```python
from build123d import *

# Parameters (mm, degrees)
SKETCH1_W                 = 175
SKETCH1_H                 = 110
BOSS_EXTRUDE1_DEPTH       = 10
SKETCH3_W                 = 30
SKETCH3_H                 = 15
BOSS_EXTRUDE2_DEPTH       = 40
M3X0_5_TAPPED_HOLE1_D     = 2.5
M3X0_5_TAPPED_HOLE1_DEPTH = 7.5
M3X0_5_TAPPED_HOLE1_TIP   = 0.751075774


with BuildPart() as part:
    # Sketch1 → Boss-Extrude1 (new body)
    with BuildSketch(Plane(origin=(0, 0, 0), x_dir=(1, 0, 0), z_dir=(0, 1, 0))):
        with Locations((87.5, 55)):
            Rectangle(SKETCH1_W, SKETCH1_H)
    extrude(amount=BOSS_EXTRUDE1_DEPTH)

    # Sketch3 → Boss-Extrude2 (add)
    with BuildSketch(Plane(origin=(0, 10, 0), x_dir=(1, 0, 0), z_dir=(0, 1, 0))):
        with Locations((55, 7.5)):
            Rectangle(SKETCH3_W, SKETCH3_H)
        with Locations((55, 102.5)):
            Rectangle(SKETCH3_W, SKETCH3_H)
    extrude(amount=BOSS_EXTRUDE2_DEPTH)

    # M3x0.5 Tapped Hole1
    with Locations(Plane(origin=(0, 50, 0), x_dir=(-1, 0, 0), z_dir=(0, 1, 0))):
        with Locations((-45, -7.5), (-65, -7.5), (-45, -102.5), (-65, -102.5)):
            Hole(M3X0_5_TAPPED_HOLE1_D / 2, depth=M3X0_5_TAPPED_HOLE1_DEPTH)
            with Locations((0, 0, -(M3X0_5_TAPPED_HOLE1_DEPTH + M3X0_5_TAPPED_HOLE1_TIP / 2))):  # 118° drill point
                Cone(0, M3X0_5_TAPPED_HOLE1_D / 2, M3X0_5_TAPPED_HOLE1_TIP, mode=Mode.SUBTRACT)


solid = part.part
```
Here's how the part is built. I have some questions about the finished solid (model axes, mm). A direction names the side the tool comes from. Coordinates: 2 decimals unless noted, no trailing zeros. Write each loop counter-clockwise with the first axis right and the second up, starting at its lowest first coordinate (ties: lowest second). Pieces come first, ordered by that corner, then holes. Notation, with made-up numbers: M 57,59 L 70,59 A27 ccw 70,80 Z; hole C -6,21.5 d4. An arc over 180 degrees is marked long. Answer as CSV lines item,"result". Start each with the question number.
Q1. Suppose I cut it at C-C, the plane z = -62.5. List the corners of the cut face in (x, y) for me, then the cut area to 3 significant figures.
Q2. Suppose I cut it at A-A, the plane y = 31. List the corners of the cut face in (x, z) for me.
Q3. Suppose I cut it at B-B, the plane y = 46.5. List the corners of the cut face in (x, z) for me.
Q4. For faces 5 (the flat face through (70, 30, -7)), 6 (the flat face through (55, 30, -95)), 7 (the flat face through (40, 30, -102)), which set-ups out of +Z, -Z, +X, -X, +Y, -Y let a thin tool reach every point of the face, with its end or its side?
Q5. Will these pins go through, and if not, where does the flat tip stop? pin 1 Ø1.5 at (x, z) = (65, -102.5) entering from +Y; pin 2 Ø16.5 at (y, z) = (36.5, -5.5) entering from +X; pin 3 Ø16.5 at (y, z) = (25.5, -100.5) entering from -X.
Q6. If we mould it in two halves opening along Z, with no side actions, what happens to faces 1 (the flat face through (55, 30, -15)), 2 (the flat face through (67, 14, 0)), 3 (the flat face through (0, 5, -54)), 4 (the flat face through (67, 14, -110))? For each: pulls with the +Z half, pulls with the -Z half, needs draft (parallel to the pull), parting line crosses it, or undercut.
Q7. Suppose I cut it at D-D, the plane x = 158. List the corners of the cut face in (y, z) for me, then the cut area to 3 significant figures.
Q8. I need wall thicknesses on probe 1 along X at (y, z) = (47.5, -7.5); probe 2 along Z at (x, y) = (65, 48); probe 3 along X at (y, z) = (44, -7). Which ranges of each line are inside material? Lowest first, please. Write a range as [from, to].
Entries:
1,outline,"M 0,0 L 175,0 L 175,10 L 0,10 Z"
1,area,"1,750 mm²"
2,outline,"M 40,-110 L 70,-110 L 70,-95 L 40,-95 Z; M 40,-15 L 70,-15 L 70,0 L 40,0 Z"
3,outline,"M 40,-110 L 70,-110 L 70,-95 L 40,-95 Z; M 40,-15 L 70,-15 L 70,0 L 40,0 Z; hole C 45,-102.5 d2.5; hole C 45,-7.5 d2.5; hole C 65,-102.5 d2.5; hole C 65,-7.5 d2.5"
4,face 5,"+Z, -Z, +X, +Y"
4,face 6,"+X, -X, +Y"
4,face 7,"+Z, -Z, -X, +Y"
5,pin 1,"stops at y = 42.2"
5,pin 2,"stops at x = 70"
5,pin 3,"stops at x = 40"
6,face 1,"undercut"
6,face 2,"pulls with the +Z half"
6,face 3,"needs draft"
6,face 4,"pulls with the -Z half"
7,outline,"M 0,-110 L 10,-110 L 10,0 L 0,0 Z"
7,area,"1,100 mm²"
8,probe 1,"x = [40, 43.75], [46.25, 63.75], [66.25, 70]"
8,probe 2,"z = [-110, -103.75], [-101.25, -95], [-15, -8.75], [-6.25, 0]"
8,probe 3,"x = [40, 43.85], [46.15, 63.85], [66.15, 70]"
